Autodesk Inventor part; units mm, degrees
ref_plane "YZ Plane" through (0, 0, 0) normal (1, 0, 0) x (0, 1, 0)
ref_plane "XZ Plane" through (0, 0, 0) normal (0, 1, 0) x (-1, 0, 0)
ref_plane "XY Plane" through (0, 0, 0) normal (0, 0, 1) x (1, 0, 0)
sketch "Sketch5" plane through (0, 0, 0) normal (0, 0, 1) x (1, 0, 0)
  line L0 (-15, 15) -> (15, 15) construction
  line L1 (15, 15) -> (15, -15) construction
  line L2 (15, -15) -> (-15, -15) construction
  line L3 (-15, -15) -> (-15, 15) construction
  line L4 (-15, 15) -> (15, -15) construction
  line L5 (15, 15) -> (-15, -15) construction
  circle A0 centre (-15, 15) radius 2
  circle A1 centre (15, 15) radius 2
  circle A2 centre (15, -15) radius 2
  circle A3 centre (-15, -15) radius 2
  line L6 (-15, 20) -> (15, 20)
  line L7 (20, 15) -> (20, -15)
  line L8 (15, -20) -> (-15, -20)
  line L9 (-20, -15) -> (-20, 15)
  line L10 (-20, 20) -> (20, -20) construction
  line L11 (20, 20) -> (-20, -20) construction
  arc A4 (20, 15) -> (15, 20) centre (15, 15) ccw
  arc A5 (15, -20) -> (20, -15) centre (15, -15) ccw
  arc A6 (-20, -15) -> (-15, -20) centre (-15, -15) ccw
  arc A7 (-15, 20) -> (-20, 15) centre (-15, 15) ccw
  point P0 (0, 0)
  dimension "d16" = 4
  dimension "d17" = 30
  dimension "d18" = 40
  dimension "d20" = 5
extrude "Extrusion5" add sketch "Sketch5" along normal blind 10
sketch "Sketch6" plane through (0, 0, 10) normal (0, 0, 1) x (1, 0, 0)
  line L0 (-15, -20) -> (15, -20)
  line L1 (-6, 20) -> (6, 20)
  line L2 (6, 20) -> (6, -20)
  line L3 (6, -20) -> (-6, -20)
  line L4 (-6, -20) -> (-6, 20)
  line L5 (-6, 20) -> (6, -20) construction
  line L6 (6, 20) -> (-6, -20) construction
  point P0 (0, 0)
  dimension "d23" = 12
extrude "Extrusion6" add sketch "Sketch6" along normal blind 40
fillet "Fillet2" radius 5 2 edges at (6, 0, 10) (-6, 0, 10)
sketch "Sketch7" plane through (6, -20, 50) normal (1, 0, 0) x (0, 0, -1)
  circle A0 centre (20, 20) radius 8.5
  circle A1 centre (20, 20) radius 20
  line L0 (0, 0) -> (0, 40)
  line L1 (40, 0) -> (40, 40)
  line L2 (35, 0) -> (0, 0)
  line L3 (20, 0) -> (0, 0)
  line L4 (0, 0) -> (0, 40)
  line L5 (0, 40) -> (20, 40)
  line L6 (35, 40) -> (0, 40)
  point P0 (50, 20)
  point P1 (0, 20)
  dimension "d27" = 17
extrude "Extrusion7" cut sketch "Sketch7" against normal blind 50 contours A0 | A1 L0 L5 | L2 L0 A1
sketch "Sketch1" plane through (0, 0, 0) normal (0, 1, 0) x (-1, 0, 0)
  line L0 (27.5, 22.5) -> (-27.5, 22.5)
  line L1 (-27.5, 22.5) -> (-27.5, -22.5)
  line L2 (-27.5, -22.5) -> (27.5, -22.5)
  line L3 (27.5, -22.5) -> (27.5, 22.5)
  point P0 (0, 0)
  point P1 (27.5, 0)
  point P2 (0, -22.5)
  dimension "d0" = 45
  dimension "d1" = 55
sketch "Sketch2" plane through (0, 10, 0) normal (0, 1, 0) x (1, 0, 0)
  line L0 (-27.5, 22.5) -> (-27.5, -22.5)
  line L1 (-27.5, -22.5) -> (27.5, -22.5)
  line L2 (-27.5, 22.5) -> (-19.5, 22.5)
  line L3 (-19.5, 22.5) -> (-19.5, -22.5)
  line L4 (-19.5, -22.5) -> (-27.5, -22.5)
  line L5 (-27.5, -22.5) -> (-27.5, 22.5)
  line L6 (27.5, -22.5) -> (27.5, 22.5)
  line L7 (27.5, 22.5) -> (19.5, 22.5)
  line L8 (19.5, 22.5) -> (19.5, -22.5)
  line L9 (19.5, -22.5) -> (27.5, -22.5)
  line L10 (27.5, -22.5) -> (27.5, 22.5)
  point P0 (0, 0)
  dimension "d4" = 8
  dimension "d5" = 8
sketch "Sketch4" plane through (0, 0, 0) normal (0, -1, 0) x (1, 0, 0)
  line L0 (15, 15) -> (-15, 15) construction
  line L1 (-15, 15) -> (-15, -15) construction
  line L2 (-15, -15) -> (15, -15) construction
  line L3 (15, -15) -> (15, 15) construction
  line L4 (15, 15) -> (-15, -15) construction
  line L5 (-15, 15) -> (15, -15) construction
  circle A0 centre (15, -15) radius 2
  circle A1 centre (-15, -15) radius 2
  circle A2 centre (-15, 15) radius 2
  circle A3 centre (15, 15) radius 2
  point P0 (0, 0)
  dimension "d12" = 30
  dimension "d13" = 4
sketch "Sketch3" plane through (27.5, 0, 22.5) normal (1, 0, 0) x (0, 0, -1)
  circle A0 centre (22.5, 25) radius 15
  line L0 (22.5, 25) -> (22.5, 47.5) construction
  line L1 (45, 47.5) -> (0, 47.5)
  line L2 (22.5, 25) -> (45, 25) construction
  line L3 (45, 0) -> (45, 47.5)
  point P0 (22.5, 0)
  dimension "d9" = 30
properties part number "DoubleHinger"
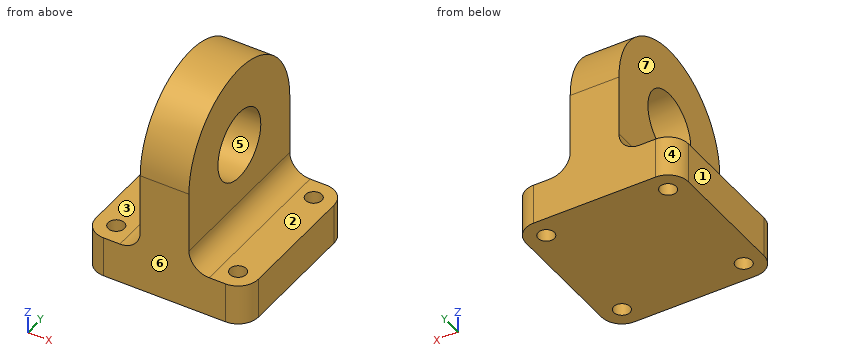
Input: part model. Units: mm. Frame: model coordinates. Face numbers are marked on the shaded views. A direction names the side the tool comes from. Coordinates: 2 decimals unless noted, no trailing zeros. Loops run counter-clockwise (first coordinate to the right, second up) from the corner with the lowest first, then second, coordinate; pieces in that order, holes last.
Q1. Cut plane C-C (z = 7.5). Output: boundary loops of the cut face in (x, y), then the cut area to 3 significant figures.
Q2. Cut plane D-D (z = 34). Output: boundary loops of the cut face in (x, y).
Q3. Draft query along Y for the marked faces 4, 5, 6 and 7. Return one class per face: +Y half, -Y half, draft (parallel to the pull), parting line (faces both ways), or undercut.
Q4. Contact query for flat-ended pins moving along their axis: pin 1 (3 mm diameter, centred on x = 15, y = 15, fed in from +Z); pin 2 (1 mm diameter, centred on x = -7, y = 13.5, fed in from -Z); pin 3 (19.5 mm diameter, centred on y = 0, z = 30, fed in from +X); pin 4 (6 mm diameter, centred on x = -10.5, y = -7.5, fed in from +Z). Output: stop coordinate, or through.
Q5. Cut plane A-A (y = 0). Output: boundary loops of the cut face in (x, z).
Q6. Material intervals for line 1 (Y direction, x = -15, z = 7); line 2 (Y direction, x = -0.5, z = 30); line 3 (Z direction, x = -2, y = 5), sorted ascending.
Q7. Cut plane B-B (x = -0.5). Output: boundary loops of the cut face in (y, z).
Q8. Set-up query: the marked faces 1, 2 and 3. Return all of +Z, -Z, +X, -X, +Y, -Y with unobstructed straight access to the full face (end or side cutting, diameter ignored); none if empty.
Working result:
1. outline: (-20, -15) arc R5 ccw to (-15, -20) - (15, -20) arc R5 ccw to (20, -15) - (20, 15) arc R5 ccw to (15, 20) - (-15, 20) arc R5 ccw to (-20, 15) - close; hole circle Ø4 at (-15, -15); hole circle Ø4 at (-15, 15); hole circle Ø4 at (15, -15); hole circle Ø4 at (15, 15)
1. area: 1,530 mm2
2. outline: (-6, -19.6) - (6, -19.6) - (6, -7.5) - (-6, -7.5) - close; (-6, 7.5) - (6, 7.5) - (6, 19.6) - (-6, 19.6) - close
3. face 4: +Y half
3. face 5: undercut
3. face 6: -Y half
3. face 7: draft
4. pin 1: passes through
4. pin 2: stops at z = 0
4. pin 3: stops at x = 6
4. pin 4: stops at z = 11.43
5. outline: (-20, 0) - (20, 0) - (20, 10) - (11, 10) arc R5 cw to (6, 15) - (6, 21.5) - (-6, 21.5) - (-6, 15) arc R5 cw to (-11, 10) - (-20, 10) - close; (-6, 38.5) - (6, 38.5) - (6, 50) - (-6, 50) - close
6. line 1: y = -20 to -17, -13 to 13, 17 to 20
6. line 2: y = -20 to -8.5, 8.5 to 20
6. line 3: z = 0 to 23.13, 36.87 to 49.36
7. outline: (-20, 0) - (20, 0) - (20, 30) arc R20 ccw to (-20, 30) - close; hole circle Ø17 at (0, 30)
8. face 1: +Z, -Z, -X, +Y, -Y
8. face 2: +Z, +X, +Y, -Y
8. face 3: +Z, -X, +Y, -Y
